Check sheet for the modelled part. Datum: model origin and axes. Units: mm. A direction names the side the tool comes from. Give positions to 0.01 mm unless a question says otherwise; leave off trailing zeros. Order: outer loops, then holes, each group sorted by start corner. A loop starts at its lowest first (then second) coordinate and runs counter-clockwise, first axis right, second up.
```python
from build123d import *

# Parameters (mm, degrees)
SKETCH1_W           = 55
SKETCH1_H           = 55
BOSS_EXTRUDE1_DEPTH = 30
SKETCH4_W           = 41
SKETCH4_H           = 16
CUT_EXTRUDE1_DEPTH  = 69.419660917
SKETCH5_W           = 16
SKETCH5_H           = 41
CUT_EXTRUDE2_DEPTH  = 60
SKETCH7_R           = 21.25
CUT_EXTRUDE3_DEPTH  = 4
SKETCH8_R           = 15
CUT_EXTRUDE4_DEPTH  = 50
SKETCH9_R           = 1.6
CUT_EXTRUDE5_DEPTH  = 10
SKETCH11_R          = 2.125
CUT_EXTRUDE6_DEPTH  = 10
FILLET2_R           = 5


with BuildPart() as part:
    # Sketch1 → Boss-Extrude1 (new body)
    with BuildSketch(Plane.XY):
        Rectangle(SKETCH1_W, SKETCH1_H)
    extrude(amount=BOSS_EXTRUDE1_DEPTH)

    # Sketch4 → Cut-Extrude1 (cut, through all)
    with BuildSketch(Plane(origin=(0, 27.5, 0), x_dir=(1, 0, 0), z_dir=(0, 1, 0))):
        with Locations((0, -15)):
            Rectangle(SKETCH4_W, SKETCH4_H)
    extrude(amount=-CUT_EXTRUDE1_DEPTH, mode=Mode.SUBTRACT)

    # Sketch5 → Cut-Extrude2 (cut)
    with BuildSketch(Plane(origin=(27.5, 0, 0), x_dir=(0, 0, -1), z_dir=(1, 0, 0))):
        with Locations((-15, 0)):
            Rectangle(SKETCH5_W, SKETCH5_H)
    extrude(amount=-CUT_EXTRUDE2_DEPTH, mode=Mode.SUBTRACT)

    # Sketch7 → Cut-Extrude3 (cut)
    with BuildSketch(Plane.XY.offset(30)):
        Circle(SKETCH7_R)
    extrude(amount=-CUT_EXTRUDE3_DEPTH, mode=Mode.SUBTRACT)

    # Sketch8 → Cut-Extrude4 (cut)
    with BuildSketch(Plane.XY.offset(26)):
        Circle(SKETCH8_R)
    extrude(amount=-CUT_EXTRUDE4_DEPTH, mode=Mode.SUBTRACT)

    # Sketch9 → Cut-Extrude5 (cut)
    with BuildSketch(Plane.XY.offset(26)):
        with Locations((0, 17.5)):
            Circle(SKETCH9_R)
        with Locations((17.5, 0)):
            Circle(SKETCH9_R)
        with Locations((0, -17.5)):
            Circle(SKETCH9_R)
        with Locations((-17.5, 0)):
            Circle(SKETCH9_R)
    extrude(amount=-CUT_EXTRUDE5_DEPTH, mode=Mode.SUBTRACT)

    # Sketch11 → Cut-Extrude6 (cut)
    with BuildSketch(Plane(origin=(0, 27.5, 0), x_dir=(1, 0, 0), z_dir=(0, 1, 0))):
        with Locations(Location((-24, -15, 0), (0, 0, 180))):
            Circle(SKETCH11_R)
        with Locations(Location((24, -15, 0), (0, 0, 180))):
            Circle(SKETCH11_R)
    extrude(amount=-CUT_EXTRUDE6_DEPTH, mode=Mode.SUBTRACT)

    # Fillet2
    fillet2_edges = [part.edges().sort_by_distance(p)[0] for p in [
        (0, 27.5, 0),
        (27.5, 0, 0),
        (0, -27.5, 0),
        (-27.5, 0, 0),
    ]]
    fillet(fillet2_edges, radius=FILLET2_R)


solid = part.part
```
Q1. Sectioned sample at C-C, the plane x = -4.5. Record the cut outline in (y, z), plus the area to 3 significant figures.
Q2. Sectioned sample at A-A, the plane z = 15. Record the cut outline in (x, y) (3 decimals).
Q3. Material ranges on line 1 (Y direction, x = 0, z = 24.2); line 2 (X direction, y = 25.5, z = 22.25); line 3 (Z direction, x = 14.5, y = 21), recorded low to high.
Q4. Sectioned sample at D-D, the plane x = -17.5. Record the cut outline in (y, z), plus the area to 3 significant figures.
Q5. Tool access check on faces 4 (the flat face through (-24, -20.5, 15)), 5 (the flat face through (13, -13, 23)), 6 (the cylindrical face through (26.123, 24.049, 15.093)), 7 (the cylindrical face through (-19.1, 0.07, 24.52)), 8 (the flat face through (27.5, 0, 26)). Record the directions out of +Z, -Z, +X, -X, +Y, -Y that give a thin tool (end or side, any length) a straight path to the whole face; none if there is none.
Q6. Draft check along Y on faces 1 (the flat face through (0, -27.5, 26)), 2 (the cylindrical face through (15.9, 0.07, 24.52)), 3 (the cylindrical face through (0.39, 26, 1.43)). Enter one of: pulls with the +Y half, pulls with the -Y half, needs draft (parallel to the pull), parting line crosses it, or undercut.
Q7. Go/stop test with flat-tipped pins: P1, Ø6, axis at x = -15, y = -5, coming from the +Z side; P2, Ø1.9, axis at x = 0, y = 17.5, coming from the +Z side; P3, Ø4, axis at x = 24, z = 15, coming from the +Y side. Record where each tip stops, or that it passes through.
Q8. Sectioned sample at B-B, the plane y = 12. Record the cut outline in (x, z), plus the area to 3 significant figures.
Filled in:
1. outline: (-27.5, 5) arc R5 ccw to (-22.5, 0) - (-14.31, 0) - (-14.31, 7) - (-27.5, 7) - close; (-27.5, 23) - (-14.31, 23) - (-14.31, 26) - (-20.77, 26) - (-20.77, 30) - (-27.5, 30) - close; (14.31, 0) - (22.5, 0) arc R5 ccw to (27.5, 5) - (27.5, 7) - (14.31, 7) - close; (14.31, 23) - (27.5, 23) - (27.5, 30) - (20.77, 30) - (20.77, 26) - (14.31, 26) - close
1. area: 307 mm2
2. outline: (-27.5, -27.5) - (-20.5, -27.5) - (-20.5, -20.5) - (-27.5, -20.5) - close; (-27.5, 20.5) - (-26.125, 20.5) - (-26.125, 27.5) - (-27.5, 27.5) - close; (-21.875, 20.5) - (-20.5, 20.5) - (-20.5, 27.5) - (-21.875, 27.5) - close; (20.5, -27.5) - (27.5, -27.5) - (27.5, -20.5) - (20.5, -20.5) - close; (20.5, 20.5) - (21.875, 20.5) - (21.875, 27.5) - (20.5, 27.5) - close; (26.125, 20.5) - (27.5, 20.5) - (27.5, 27.5) - (26.125, 27.5) - close
3. line 1: y = -27.5 to -19.1, -15.9 to -15, 15 to 15.9, 19.1 to 27.5
3. line 2: x = -27.5 to -20.5, 20.5 to 27.5
3. line 3: z = 0 to 7, 23 to 30
4. outline: (-27.5, 5) arc R5 ccw to (-22.5, 0) - (22.5, 0) arc R5 ccw to (27.5, 5) - (27.5, 7) - (-27.5, 7) - close; (-27.5, 23) - (-1.6, 23) - (-1.6, 26) - (-12.05, 26) - (-12.05, 30) - (-27.5, 30) - close; (1.6, 23) - (27.5, 23) - (27.5, 30) - (12.05, 30) - (12.05, 26) - (1.6, 26) - close
4. area: 653 mm2
5. face 4: +X, -X
5. face 5: none
5. face 6: +Y
5. face 7: +Z
5. face 8: +Z, -Z, +X, +Y, -Y
6. face 1: pulls with the -Y half
6. face 2: undercut
6. face 3: pulls with the +Y half
7. P1: stops at z = 26
7. P2: stops at z = 7
7. P3: stops at y = -20.5
8. outline: (-27.5, 5) arc R5 ccw to (-22.5, 0) - (-9, 0) - (-9, 7) - (-27.5, 7) - close; (-27.5, 23) - (-9, 23) - (-9, 26) - (-17.54, 26) - (-17.54, 30) - (-27.5, 30) - close; (9, 0) - (22.5, 0) arc R5 ccw to (27.5, 5) - (27.5, 7) - (9, 7) - close; (9, 23) - (27.5, 23) - (27.5, 30) - (17.54, 30) - (17.54, 26) - (9, 26) - close
8. area: 439 mm2
